Here's how the part is built. I have some questions about the finished solid (model axes, mm). Face numbers are marked on the shaded views. A direction names the side the tool comes from. Give positions to 0.01 mm unless a question says otherwise; leave off trailing zeros. Loops run counter-clockwise (first coordinate to the right, second up) from the corner with the lowest first, then second, coordinate; pieces in that order, holes last. Notation, with made-up numbers: M 3,-13 L 9,-13 A16 ccw 9,-4 Z; hole C 48,8.5 d11. An arc over 180 degrees is marked long. Write item = value, one per line. Start each with the question number.
Autodesk Inventor part; units mm, degrees
ref_plane "YZ Plane" through (0, 0, 0) normal (1, 0, 0) x (0, 1, 0)
ref_plane "XZ Plane" through (0, 0, 0) normal (0, 1, 0) x (-1, 0, 0)
ref_plane "XY Plane" through (0, 0, 0) normal (0, 0, 1) x (1, 0, 0)
sketch "Sketch1" plane through (0, 0, 0) normal (0, 0, 1) x (1, 0, 0)
  line L0 (0, 35.9415) -> (0, -22.75) construction
  line L1 (5, 30) -> (15, 30)
  line L2 (15, 30) -> (15, -30)
  line L3 (15, -30) -> (5, -30)
  line L4 (5, -30) -> (5, 30)
  circle A0 centre (10, 25) radius 2.25
  circle A1 centre (10, -25) radius 2.25
  line L5 (-5, 22.5) -> (5, 22.5)
  line L6 (5, 22.5) -> (5, -22.5)
  line L7 (5, -22.5) -> (-5, -22.5)
  line L8 (-5, -22.5) -> (-5, 22.5)
  line L9 (-5, 22.5) -> (5, 22.5)
  line L10 (5, 22.5) -> (5, 16.5)
  line L11 (5, 16.5) -> (-5, 16.5)
  line L12 (-5, 16.5) -> (-5, 22.5)
  line L13 (-5, -22.5) -> (5, -22.5)
  line L14 (5, -22.5) -> (5, -16.5)
  line L15 (5, -16.5) -> (-5, -16.5)
  line L16 (-5, -16.5) -> (-5, -22.5)
  line L17 (-5, 3) -> (5, 3)
  line L18 (5, 3) -> (5, -3)
  line L19 (5, -3) -> (-5, -3)
  line L20 (-5, -3) -> (-5, 3)
  point P0 (0, 0)
  point P1 (15, 0)
  point P2 (5, 0)
  point P3 (0, 22.5)
  point P4 (5, 0)
  point P5 (5, 0)
  dimension "d28" = 60
  dimension "d29" = 4.5
  dimension "d30" = 4.5
  dimension "d31" = 5
  dimension "d32" = 5
  dimension "d33" = 10
  dimension "d36" = 10
  dimension "d37" = 45
  dimension "d38" = 5
  dimension "d39" = 5
  dimension "d42" = 6
  dimension "d43" = 6
  dimension "d44" = 6
extrude "Extrusion3" add sketch "Sketch1" along normal blind 0.6 contours L4 L11 L8 L5 | L4 L17 L8 L11 | L4 L19 L8 L17 | L7 L8 L15 L4 | L4 L15 L8 L19
extrude "Extrusion4" add sketch "Sketch1" along normal blind 0.6 contours L1 L2 L3 L4
mirror "Mirror1" about plane through (0, 0, 0) normal (1, 0, 0) of "Extrusion4"
extrude "Extrusion5" add sketch "Sketch1" along normal blind 1.8 contours L1 L2 L3 L4
extrude "Extrusion6" add sketch "Sketch1" along normal blind 1.8 contours L4 L11 L8 L5 | L4 L19 L8 L17 | L7 L8 L15 L4
mirror "Mirror2" about plane through (0, 0, 0) normal (1, 0, 0) of "Extrusion5", "Extrusion6"
equation "\"d29\" = screw"
equation "\"d30\" = screw"
properties part number "FoldLink" material "Rubber, Silicone"
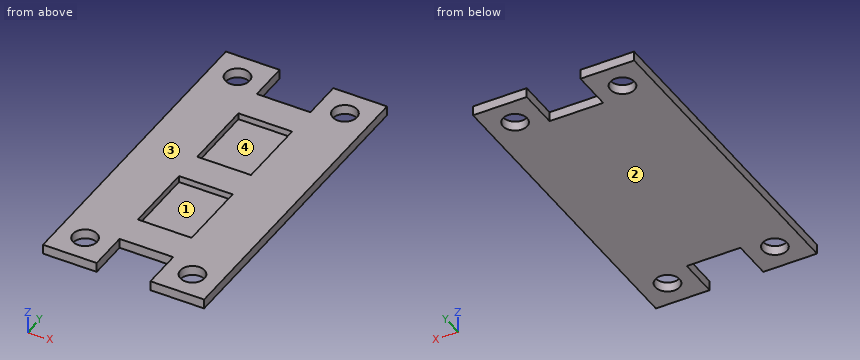
Q1. If we section it at C-C, the plane y = -25: List the corners of the cut face in (x, z) for me, then the cut area to 3 significant figures.
Q2. If I drill on line 1 along Y through (x, z) = (10.25, 0.35); line 2 along Y through (x, z) = (4.5, 1.3); line 3 along X through (y, z) = (-26.5, 0.7), over which ranges is the centre line in solid material (lowest first)?
Q3. We'd pull the mould along Y, two halves only. Please class the marked faces 3 and 4: pulls with the +Y half, pulls with the -Y half, needs draft (parallel to the pull), parting line crosses it, or undercut.
Q4. If we section it at D-D, the plane y = -10.5: List the corners of the cut face in (x, z) for me, then the cut area to 3 significant figures.
Q5. If we section it at A-A, the plane x = 10: List the corners of the cut face in (y, z) for me.
Q6. Will this pin go through, and if not, where does the flat tip stop? pin 1 (0.6 mm diameter, centred on x = -2, z = 1.5, fed in from -Y).
Q7. On a 3-axis mill with a long thin cutter (end or side, diameter ignored), from which of +Z, -Z, +X, -X, +Y, -Y can I reach the whole of each face in a straight line? I mean the marked faces 1 and 2. Say none if no direction works.
Q8. If we section it at B-B, the plane z = 1.5: List the corners of the cut face in (x, y) for me, then the cut area to 3 significant figures.
Resolved:
q1.outline = M -15,0 L -12.25,0 L -12.25,1.8 L -15,1.8 Z; M -7.75,0 L -5,0 L -5,1.8 L -7.75,1.8 Z; M 5,0 L 7.75,0 L 7.75,1.8 L 5,1.8 Z; M 12.25,0 L 15,0 L 15,1.8 L 12.25,1.8 Z
q1.area = 19.8 mm²
q2.line_1 = -30 to -27.24, -22.76 to 22.76, 27.24 to 30
q2.line_2 = -22.5 to -16.5, -3 to 3, 16.5 to 22.5
q2.line_3 = -15 to -11.68, -8.32 to -5, 5 to 8.32, 11.68 to 15
q3.face_3 = needs draft
q3.face_4 = undercut
q4.outline = M -15,0 L 15,0 L 15,1.8 L 5,1.8 L 5,0.6 L -5,0.6 L -5,1.8 L -15,1.8 Z
q4.area = 42.0 mm²
q5.outline = M -30,0 L -27.25,0 L -27.25,1.8 L -30,1.8 Z; M -22.75,0 L 22.75,0 L 22.75,1.8 L -22.75,1.8 Z; M 27.25,0 L 30,0 L 30,1.8 L 27.25,1.8 Z
q6.pin_1 = -22.5
q7.face_1 = +Z
q7.face_2 = -Z, +X, -X, +Y, -Y
q8.outline = M -15,-30 L -5,-30 L -5,-22.5 L 5,-22.5 L 5,-30 L 15,-30 L 15,30 L 5,30 L 5,22.5 L -5,22.5 L -5,30 L -15,30 Z; hole C -10,-25 d4.5; hole C -10,25 d4.5; hole M -5,-16.5 L 5,-16.5 L 5,-3 L -5,-3 Z; hole M -5,3 L 5,3 L 5,16.5 L -5,16.5 Z; hole C 10,-25 d4.5; hole C 10,25 d4.5
q8.area = 1,320 mm²
